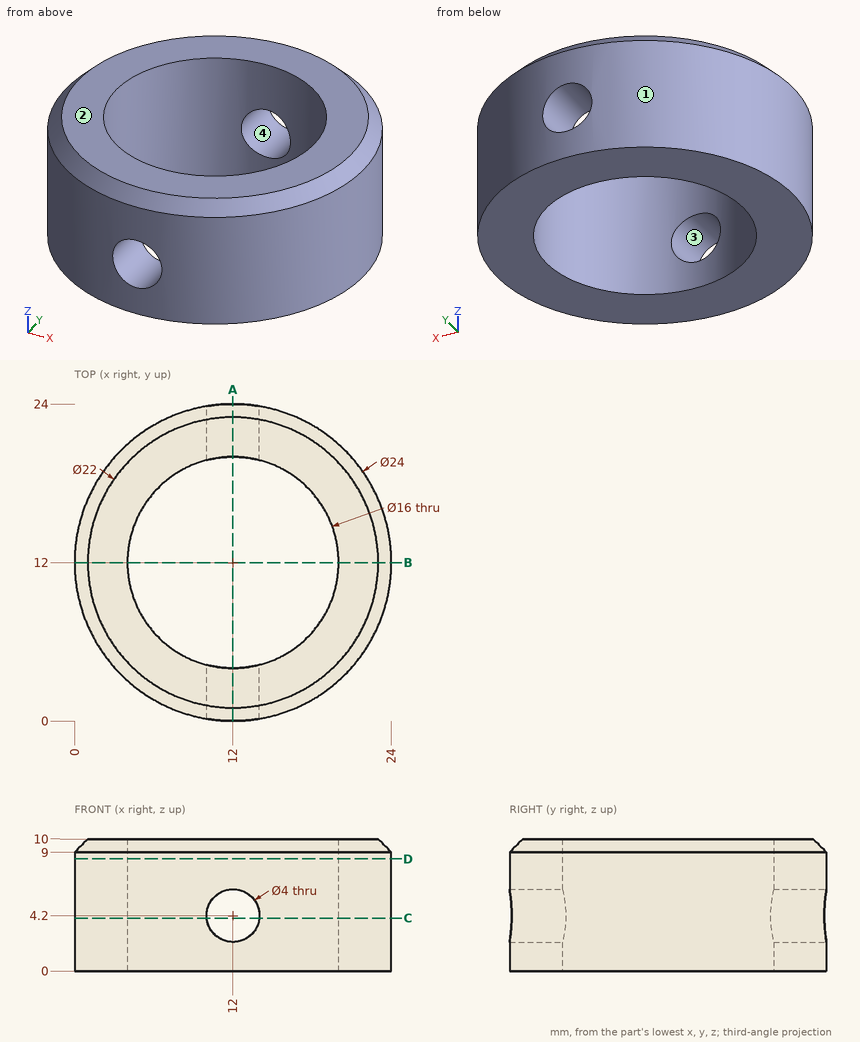
Drawing for the job (mm, zero at the part's lowest x, y, z). Give positions to 0.01 mm unless a question says otherwise; leave off trailing zeros. Order: outer loops, then holes, each group sorted by start corner. A loop starts at its lowest first (then second) coordinate and runs counter-clockwise, first axis right, second up. Notation, with made-up numbers: M 81.5,-7.5 L 100.5,-7.5 A22 ccw 100.5,31.5 Z; hole C -20.5,-11.75 d6. An arc over 180 degrees is marked long. Put each result on its own line as item: value. Start each with the question number.
(1) Flat gauge pins, fed straight in: pin 1 Ø6 at (x, z) = (9, 6) entering from -Y; pin 2 Ø3.5 at (x, z) = (12, 4.2) entering from +Y; pin 3 Ø1 at (x, z) = (8.5, 7.5) entering from -Y. Where does each tip first touch, or does it go through?
(2) Saw through at C-C, the plane z = 4. Write the cut outline in (x, y).
(3) Drill centre lines: line 1 along X through (y, z) = (22.05, 4.2); line 2 along Y through (x, z) = (17.25, 7.5); line 3 along Z through (x, y) = (13.5, 22). Where is each one in solid material? Low to high.
(4) Saw through at A-A, the plane x = 12. Write the cut outline in (y, z), then the cut area to 3 significant figures.
(5) Mould opens along X. For the marked faces 1, 2, 3 and 4 say: +X half, -X half, draft (parallel to the pull), parting line (faces both ways), or undercut.
(6) Saw through at B-B, the plane y = 12. Write the cut outline in (x, z).
(7) Saw through at D-D, the plane z = 8.5. Write the cut outline in (x, y).
Check result:
1. pin 1: stops at y = 0
1. pin 2: passes through
1. pin 3: stops at y = 0.38
2. outline: M 10.01,0.17 L 10.01,4.25 A8 cw 10.01,19.75 L 10.01,23.83 A12 ccw Z; M 13.99,0.17 A12 ccw 13.99,23.83 L 13.99,19.75 A8 cw 13.99,4.25 Z
3. line 1: x = 5.44 to 10, 14 to 18.56
3. line 2: y = 1.21 to 5.96, 18.04 to 22.79
3. line 3: z = 0 to 2.88, 5.52 to 10
4. outline: M 0,0 L 4,0 L 4,2.2 L 0,2.2 Z; M 0,6.2 L 4,6.2 L 4,10 L 1,10 L 0,9 Z; M 20,0 L 24,0 L 24,2.2 L 20,2.2 Z; M 20,6.2 L 24,6.2 L 24,9 L 23,10 L 20,10 Z
4. area: 47.0 mm2
5. face 1: parting line
5. face 2: draft
5. face 3: undercut
5. face 4: undercut
6. outline: M 0,0 L 4,0 L 4,10 L 1,10 L 0,9 Z; M 20,0 L 24,0 L 24,9 L 23,10 L 20,10 Z
7. outline: C 12,12 d24; hole C 12,12 d16
